from build123d import *

# Parameters (mm, degrees)
BOSS_EXTRUDE1_DEPTH = 7.5
SKETCH2_R           = 1.6
CUT_EXTRUDE1_DEPTH  = 15
SKETCH3_R           = 1.6
CUT_EXTRUDE2_DEPTH  = 15


with BuildPart() as part:
    # Sketch1 → Boss-Extrude1 (new, symmetric)
    with BuildSketch(Plane.XY):
        Polygon((0, 0), (-15, 0), (-15, 3), (3, 3), (3, -7), (0, -7), align=None)
    extrude(amount=BOSS_EXTRUDE1_DEPTH, both=True)

    # Sketch2 → Cut-Extrude1 (cut)
    with BuildSketch(Plane(origin=(0, 3, 0), x_dir=(1, 0, 0), z_dir=(0, 1, 0))):
        with Locations(Location((-11, 3.5, 0), (0, 0, 180))):
            Circle(SKETCH2_R)
        with Locations(Location((-11, -3.5, 0), (0, 0, 180))):
            Circle(SKETCH2_R)
    extrude(amount=-CUT_EXTRUDE1_DEPTH, mode=Mode.SUBTRACT)

    # Sketch3 → Cut-Extrude2 (cut)
    with BuildSketch(Plane(origin=(3, 0, 0), x_dir=(0, 0, -1), z_dir=(1, 0, 0))):
        with Locations((-3.5, -4)):
            Circle(SKETCH3_R)
        with Locations((3.5, -4)):
            Circle(SKETCH3_R)
    extrude(amount=-CUT_EXTRUDE2_DEPTH, mode=Mode.SUBTRACT)


solid = part.part
Here's how the part is built. I have some questions about the finished solid (model axes, mm). A direction names the side the tool comes from. Coordinates: 2 decimals unless noted, no trailing zeros. Loops run counter-clockwise (first coordinate to the right, second up) from the corner with the lowest first, then second, coordinate; pieces in that order, holes last.
1. If we mould it in two halves opening along X, with no side actions, what happens to faces 3 (the flat face through (-3.9, 0.3, 7.5)), 4 (the cylindrical face through (-9.4, 1.52, -3.43)), 5 (the cylindrical face through (-9.4, 1.52, 3.57)), 6 (the flat face through (0, -4, 0))? For each: pulls with the +X half, pulls with the -X half, needs draft (parallel to the pull), parting line crosses it, or undercut.
2. Imagine slicing it at B-B, the plane z = -3.5. Please give me the cut outline in (x, y).
3. For faces 1 (the flat face through (3, -2, 0)), 2 (the flat face through (-7, 0, 0)), which set-ups out of +Z, -Z, +X, -X, +Y, -Y let a thin tool reach every point of the face, with its end or its side?
4. Imagine slicing it at A-A, the plane x = -11. Please give me the cut outline in (y, z), and give its area (3 significant figures).
5. Imagine slicing it at D-D, the plane y = 2. Please give me the cut outline in (x, z).
6. I need wall thicknesses on L1, parallel to Z at x = -11, y = 2.25; L2, parallel to Y at x = 1.4, z = 3.5; L3, parallel to Z at x = 2, y = -5. Which ranges of each line are inside material? Lowest first, please.
7. For P1, Ø7.5, axis at x = -7.5, z = 1.5, coming from the -Y side; P2, Ø3, axis at x = -11, z = 3.5, coming from the +Y side; P3, Ø5, axis at y = -4, z = -3.5, coming from the -X side, each with a flat end and sliding along its axis, tell me the tip position at first contact or that it passes through.
Taken from the geometry:
1. face 3: needs draft
1. face 4: undercut
1. face 5: undercut
1. face 6: pulls with the -X half
2. outline: (-15, 0) - (-12.6, 0) - (-12.6, 3) - (-15, 3) - close; (-9.4, 0) - (0, 0) - (0, -2.4) - (3, -2.4) - (3, 3) - (-9.4, 3) - close; (0, -7) - (3, -7) - (3, -5.6) - (0, -5.6) - close
3. face 1: +Z, -Z, +X, +Y, -Y
3. face 2: +Z, -Z, -X, -Y
4. outline: (0, -7.5) - (3, -7.5) - (3, -5.1) - (0, -5.1) - close; (0, -1.9) - (3, -1.9) - (3, 1.9) - (0, 1.9) - close; (0, 5.1) - (3, 5.1) - (3, 7.5) - (0, 7.5) - close
4. area: 25.8 mm2
5. outline: (-15, -7.5) - (3, -7.5) - (3, 7.5) - (-15, 7.5) - close; hole circle Ø3.2 at (-11, -3.5); hole circle Ø3.2 at (-11, 3.5)
6. L1: z = -7.5 to -5.1, -1.9 to 1.9, 5.1 to 7.5
6. L2: y = -7 to -5.6, -2.4 to 3
6. L3: z = -7.5 to -4.75, -2.25 to 2.25, 4.75 to 7.5
7. P1: stops at y = 0
7. P2: passes through
7. P3: stops at x = 0
